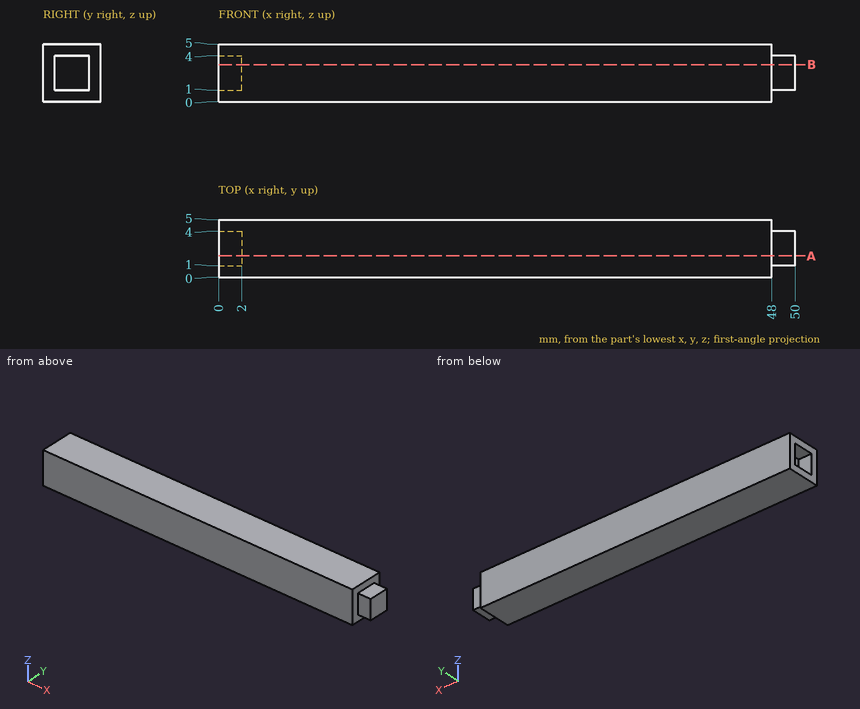
Geometry check sheet. Reference: drawing and pictorial views, mm from the part's lowest x, y, z. Coordinates: 2 decimals unless noted, no trailing zeros. Loops run counter-clockwise (first coordinate to the right, second up) from the corner with the lowest first, then second, coordinate; pieces in that order, holes last.
1) Gauge pin test, flat ends, axial feed: pin 1 (2 mm diameter, centred on x = 1.5, z = 2, fed in from -Y); pin 2 (1.5 mm diameter, centred on y = 3, z = 2, fed in from -X); pin 3 (1.6 mm diameter, centred on x = 49.5, y = 3, fed in from +Z). Record the tip position at first contact, or that the pin passes through.
2) Material ranges on probe 1 along X at (y, z) = (2.25, 4.15); probe 2 along X at (y, z) = (2.2, 3.5), recorded low to high.
3) Sectioned sample at A-A (y = 1.85). Record the boundary of the cut face in (x, z).
Check sheet entries:
1. pin 1: stops at y = 0
1. pin 2: stops at x = 2
1. pin 3: stops at z = 4
2. probe 1: x = 0 to 48
2. probe 2: x = 2 to 50
3. outline: (0, 0) - (48, 0) - (48, 1) - (50, 1) - (50, 4) - (48, 4) - (48, 5) - (0, 5) - (0, 4) - (2, 4) - (2, 1) - (0, 1) - close
